Design review of the part built by this model. Coordinates are the model's own, in mm. A direction names the side the tool comes from. Give positions to 0.01 mm unless a question says otherwise; leave off trailing zeros. Loops run counter-clockwise (first coordinate to the right, second up) from the corner with the lowest first, then second, coordinate; pieces in that order, holes last.
from build123d import *

# Parameters (mm, degrees)
F0_W     = 32
F0_H     = 100
F0_R     = 9.5
F1_DEPTH = 32
F2_R     = 11
F3_DEPTH = 32.001
F4_W     = 32
F4_H     = 2.6
F5_DEPTH = 25
F6_R     = 15.99999
F7_R     = 3
F8_DEPTH = 100.001


# Not quite as in the source:
# - a fillet or chamfer is up to 0.001 mm smaller than in the source, because OpenCascade refuses the exact size


with BuildPart() as f1:
    # F0 (on Right) → F1 (new body)
    with BuildSketch(Plane.YZ):
        Rectangle(F0_W, F0_H)
        with Locations((0, -22.4)):
            Circle(F0_R, mode=Mode.SUBTRACT)
        with Locations((0, 22.4)):
            Circle(F0_R, mode=Mode.SUBTRACT)
    extrude(amount=F1_DEPTH)

    # F2 (on face) → F3 (cut, through all)
    with BuildSketch(Plane.XZ.offset(16)):
        with Locations((16, 0)):
            Circle(F2_R)
    extrude(amount=-F3_DEPTH, mode=Mode.SUBTRACT)

    # F4 (on face) → F5 (join)
    with BuildSketch(Plane.YZ.offset(32)):
        with Locations((0, 48.7)):
            Rectangle(F4_W, F4_H)
        with Locations((0, 38.1)):
            Rectangle(F4_W, F4_H)
        with Locations((0, -38.1)):
            Rectangle(F4_W, F4_H)
        with Locations((0, -48.7)):
            Rectangle(F4_W, F4_H)
    extrude(amount=F5_DEPTH)

    # F6 (radius 16 in the source; OpenCascade refuses exactly that, so slightly less here)
    f6_edges = [f1.edges().sort_by_distance(p)[0] for p in [
        (57, -16, 48.7),
        (57, -16, 38.1),
        (57, 16, 38.1),
        (57, 16, 48.7),
        (57, 16, -48.7),
        (57, -16, -48.7),
        (57, -16, -38.1),
        (57, 16, -38.1),
    ]]
    fillet(f6_edges, radius=F6_R)

    # F7 (on face) → F8 (cut, through all)
    with BuildSketch(Plane.XY.offset(50)):
        with Locations((41, 0)):
            Circle(F7_R)
    extrude(amount=-F8_DEPTH, mode=Mode.SUBTRACT)


solid = f1.part
Q1. Wall thickness on line 1 (Z direction, x = 43, y = 10.5); line 2 (Y direction, x = 41, z = 49); line 3 (Z direction, x = 24, y = 0): over which ranges is each line inside the solid? List them lowest first.
Results:
line 1: z = -50 to -47.4, -39.4 to -36.8, 36.8 to 39.4, 47.4 to 50
line 2: y = -16 to -3, 3 to 16
line 3: z = -50 to -31.9, -12.9 to -7.55, 7.55 to 12.9, 31.9 to 50
Q2. Take a section at B-B (x = 12.5). Give the boundary of the cut face in (y, z).
Results:
outline: (-16, -50) - (16, -50) - (16, -10.43) - (-16, -10.43) - close; (-16, 10.43) - (16, 10.43) - (16, 50) - (-16, 50) - close; hole circle Ø19 at (0, -22.4); hole circle Ø19 at (0, 22.4)
Q3. Take a section at C-C (y = 1). Give the number of separate pieces and of enclosed holes in the cut face, plus the area to 3 significant figures.
Results:
separate pieces: 7
enclosed holes: 1
area: 1,810 mm2
Q4. Draft analysis for pull direction Z (two halves, no side actions). For faces 3 (the face through (26.161, -0.224, -4.213)), 4 (the face through (52.189, 11.437, -38.082)), 5 (the face through (28, 0, -50)), state which applies: pulls with the +Z half, pulls with the -Z half, needs draft (parallel to the pull), parting line crosses it, or undercut.
Results:
face 3: undercut
face 4: needs draft
face 5: pulls with the -Z half
Q5. Take a section at D-D (x = 50.5). Give the boundary of the cut face in (y, z).
Results:
outline: (-12.87, -50) - (12.87, -50) - (12.87, -47.4) - (-12.87, -47.4) - close; (-12.87, -39.4) - (12.87, -39.4) - (12.87, -36.8) - (-12.87, -36.8) - close; (-12.87, 36.8) - (12.87, 36.8) - (12.87, 39.4) - (-12.87, 39.4) - close; (-12.87, 47.4) - (12.87, 47.4) - (12.87, 50) - (-12.87, 50) - close
Q6. Take a section at A-A (z = -22.4). Give the boundary of the cut face in (x, y), plus the area to 3 significant figures.
Results:
outline: (0, -16) - (32, -16) - (32, -9.5) - (0, -9.5) - close; (0, 9.5) - (32, 9.5) - (32, 16) - (0, 16) - close
area: 416 mm2
Q7. Insertion check: pin 1 (2.5 mm diameter, centred on y = -7, z = 43, fed in from +X); pin 2 (9 mm diameter, centred on y = 7.5, z = -42, fed in from +X). Each pin has a flat end and moves straight along its axis. Give the tip position at first contact, or say it passes through.
Results:
pin 1: stops at x = 32
pin 2: stops at x = 56.54
Q8. Tool access review of faces 1 (the face through (38, 0, -38)), 2 (the face through (44.3, -0.2, 39.4)): name each direction out of +Z, -Z, +X, -X, +Y, -Y from which nothing blocks a thin tool from reaching the whole face with its end or side.
Results:
face 1: +Z, -Z
face 2: +X, +Y, -Y
